Part model, mm, in its own coordinate system. A direction names the side the tool comes from. Round coordinates to 2 decimals unless told otherwise and drop trailing zeros. Loops run counter-clockwise (first coordinate to the right, second up) from the corner with the lowest first, then second, coordinate; pieces in that order, holes last. Notation, with made-up numbers: M 14.25,59 L 31.25,59 A23 ccw 31.25,93 Z; hole C -37.5,44 d1. An arc over 180 degrees is marked long. Write each question's results on one line, items separated by ' | '.
from build123d import *

# Parameters (mm, degrees)
SKETCH2_R                                       = 7.5
BOSS_EXTRUDE1_DEPTH                             = 8
CSK_FOR_M3_FLAT_HEAD_MACHINE_SCREW2_D           = 3.2
CSK_FOR_M3_FLAT_HEAD_MACHINE_SCREW2_CSINK_D     = 8.3
CSK_FOR_M3_FLAT_HEAD_MACHINE_SCREW2_CSINK_ANGLE = 90
FILLET1_R                                       = 20
V_GROOVE_CUTOUT_FLIPPED_DEPTH                   = 3.6
SKETCH49_R                                      = 2.55
CUT_EXTRUDE3_DEPTH                              = 52.922196079
CHAMFER2_SIZE                                   = 0.4
CHAMFER2_SIZE2                                  = 1.098990968
MOVE_FACE2_BY                                   = 0.5
MOVE_FACE2_2_BY                                 = 0.5
MOVE_FACE2_3_BY                                 = 0.5
MOVE_FACE2_4_BY                                 = 0.5
MOVE_FACE2_5_BY                                 = 0.5
MOVE_FACE2_6_BY                                 = 0.5
CIRPATTERN2_COUNT                               = 3
SKETCH20_R                                      = 1.375
TOOL_WING_SCREW_HOLES_DEPTH                     = 4
FILLET17_R                                      = 2
FILLET18_R                                      = 1
SKETCH50_R                                      = 1.375
CUT_EXTRUDE4_DEPTH                              = 4


with BuildPart() as part:
    # Sketch2 → Boss-Extrude1 (new body)
    with BuildSketch(Plane.XY):
        Polygon((-18, 40), (18, 40), (18, -4.618802154), (32.810889132, -13.169872981), (27.810889132, -21.830127019), (-27.810889132, -21.830127019), (-32.810889132, -13.169872981), (-18, -4.618802154), align=None)
        Circle(SKETCH2_R, mode=Mode.SUBTRACT)
    extrude(amount=BOSS_EXTRUDE1_DEPTH)

    # CSK for M3 Flat Head Machine Screw2 (through all)
    with Locations(Plane.XY.offset(8)):
        with Locations((-25.980762114, -15), (0, 30), (25.980762114, -15)):
            CounterSinkHole(CSK_FOR_M3_FLAT_HEAD_MACHINE_SCREW2_D / 2, CSK_FOR_M3_FLAT_HEAD_MACHINE_SCREW2_CSINK_D / 2, counter_sink_angle=CSK_FOR_M3_FLAT_HEAD_MACHINE_SCREW2_CSINK_ANGLE)

    # Fillet1
    fillet1_edges = [part.edges().sort_by_distance(p)[0] for p in [
        (18, -4.618802154, 4),
        (-18, -4.618802154, 4),
    ]]
    fillet(fillet1_edges, radius=FILLET1_R)

    # Sketch47 → v-groove cutout flipped (cut)
    with BuildSketch(Plane(origin=(0, 0, 0), x_dir=(-1, 0, 0), z_dir=(0, 0, -1))):
        with BuildLine():
            Line((-3.464101615, 14), (-13.856406461, -4))
            ThreePointArc((-13.856406461, -4), (-13.856406461, -8), (-10.392304845, -10))
            Line((-10.392304845, -10), (10.392304845, -10))
            ThreePointArc((10.392304845, -10), (13.856406461, -8), (13.856406461, -4))
            Line((13.856406461, -4), (3.464101615, 14))
            ThreePointArc((3.464101615, 14), (0, 16), (-3.464101615, 14))
        make_face()
    extrude(amount=-V_GROOVE_CUTOUT_FLIPPED_DEPTH, mode=Mode.SUBTRACT)

    # Sketch49 → Cut-Extrude3 (cut, through all)
    with BuildSketch(Plane(origin=(0, 0, 3.6), x_dir=(-1, 0, 0), z_dir=(0, 0, -1))):
        with Locations((0, 12)):
            Circle(SKETCH49_R)
        with Locations((10.392304845, -6)):
            Circle(SKETCH49_R)
        with Locations((-10.392304845, -6)):
            Circle(SKETCH49_R)
    extrude(amount=-CUT_EXTRUDE3_DEPTH, mode=Mode.SUBTRACT)

    # Chamfer2
    chamfer2_edges = [part.edges().sort_by_distance(p)[0] for p in [
        (2.55, 12, 8),
        (-7.842304845, -6, 8),
        (12.942304845, -6, 8),
    ]]
    chamfer2_side = [part.faces().sort_by_distance(p)[0] for p in [
        (17.098380214, 23.464101615, 8),
    ]]
    chamfer(chamfer2_edges, length=CHAMFER2_SIZE, length2=CHAMFER2_SIZE2, reference=chamfer2_side[0])

    # Move Face2: a curved face moved inward by 0.5
    add(Solid.thicken(part.faces().sort_by_distance((-13.856406461, -8, 1.8))[0], -MOVE_FACE2_BY), mode=Mode.SUBTRACT)

    # Move Face2 2: a face moved inward by 0.5
    extrude(part.faces().sort_by_distance((0, -10, 1.8))[0], amount=MOVE_FACE2_2_BY, dir=(0, -1, 0), mode=Mode.SUBTRACT)

    # Move Face2 3: a curved face moved inward by 0.5
    add(Solid.thicken(part.faces().sort_by_distance((13.856406461, -8, 1.8))[0], -MOVE_FACE2_3_BY), mode=Mode.SUBTRACT)

    # Move Face2 4: a face moved inward by 0.5
    extrude(part.faces().sort_by_distance((8.660254038, 5, 1.8))[0], amount=MOVE_FACE2_4_BY, dir=(0.866025404, 0.5, 0), mode=Mode.SUBTRACT)

    # Move Face2 5: a curved face moved inward by 0.5
    add(Solid.thicken(part.faces().sort_by_distance((0, 16, 1.8))[0], -MOVE_FACE2_5_BY), mode=Mode.SUBTRACT)

    # Move Face2 6: a face moved inward by 0.5
    extrude(part.faces().sort_by_distance((-8.660254038, 5, 1.8))[0], amount=MOVE_FACE2_6_BY, dir=(-0.866025404, 0.5, 0), mode=Mode.SUBTRACT)

    # Sketch46 → tool ball cutout (revolve, cut)
    with BuildSketch(Plane(origin=(0, 30, 0), x_dir=(1, 0, 0), z_dir=(0, 1, 0))):
        with BuildLine():
            Line((0, 4.3), (0, -3.7))
            ThreePointArc((0, -3.7), (-4, 0.3), (0, 4.3))
        make_face()
    tool_ball_cutout = revolve(axis=Axis((0, 30, 0), (0, 0, -1)), mode=Mode.SUBTRACT)

    # CirPattern2: tool ball cutout ×3 about axis
    cirpattern2_axis = Axis((0, 0, 0), (0, 0, 1))
    for i in range(1, CIRPATTERN2_COUNT):
        add(tool_ball_cutout.rotate(cirpattern2_axis, i * 360 / CIRPATTERN2_COUNT), mode=Mode.SUBTRACT)

    # Sketch20 → Tool Wing Screw Holes (cut)
    with BuildSketch(Plane(origin=(18, 0, 0), x_dir=(0, 0, -1), z_dir=(1, 0, 0))):
        with Locations(Location((-4, 19, 0), (0, 0, 90))):
            Circle(SKETCH20_R)
        with Locations(Location((-4, 32.5, 0), (0, 0, 90))):
            Circle(SKETCH20_R)
    tool_wing_screw_holes = extrude(amount=-TOOL_WING_SCREW_HOLES_DEPTH, mode=Mode.SUBTRACT)

    # Mirror2: Tool Wing Screw Holes across plane
    add(tool_wing_screw_holes.mirror(Plane(origin=(0, 0, 0), x_dir=(0, 0, 1), z_dir=(1, 0, 0))), mode=Mode.SUBTRACT)

    # Fillet17
    fillet17_edges = [part.edges().sort_by_distance(p)[0] for p in [
        (32.810889132, -13.169872981, 4),
        (27.810889132, -21.830127019, 4),
        (-27.810889132, -21.830127019, 4),
        (-32.810889132, -13.169872981, 4),
    ]]
    fillet(fillet17_edges, radius=FILLET17_R)

    # Fillet18
    fillet18_edges = [part.edges().sort_by_distance(p)[0] for p in [
        (-18, 40, 4),
        (18, 40, 4),
    ]]
    fillet(fillet18_edges, radius=FILLET18_R)

    # Sketch50 → Cut-Extrude4 (cut)
    with BuildSketch(Plane.XZ.offset(21.830127019)):
        with Locations((-15, 4)):
            Circle(SKETCH50_R)
        with Locations((15, 4)):
            Circle(SKETCH50_R)
    extrude(amount=-CUT_EXTRUDE4_DEPTH, mode=Mode.SUBTRACT)


solid = part.part
Item 1: Band-saw the part on A-A on x = 0. Give the cut face in (y, z).
Filled sheet:
outline: M -21.83,0 L -10.5,0 L -10.5,3.6 L -7.5,3.6 L -7.5,8 L -21.83,8 Z; M 7.5,3.6 L 9.45,3.6 L 9.45,6.9 L 9.05,8 L 7.5,8 Z; M 14.55,3.6 L 16.5,3.6 L 16.5,0 L 26.01,0 A4 cw 28.4,3.37 L 28.4,5.45 L 25.85,8 L 14.95,8 L 14.55,6.9 Z; M 31.6,3.37 A4 cw 33.99,0 L 40,0 L 40,8 L 34.15,8 L 31.6,5.45 Z
Item 2: Band-saw the part on B-B on y = 0. Give the cut face in (x, z).
Filled sheet:
outline: M -19.24,0 L -12.12,0 L -12.12,3.6 L -7.5,3.6 L -7.5,8 L -19.24,8 Z; M 7.5,3.6 L 12.12,3.6 L 12.12,0 L 19.24,0 L 19.24,8 L 7.5,8 Z
Item 3: Drop flat-ended pins along their axis: P1, Ø0.8, axis at y = 18.5, z = 3.5, coming from the -X side; P2, Ø1.5, axis at y = 22, z = 1, coming from the +X side; P3, Ø6, axis at x = 17, y = -14.5, coming from the -Z side; P4, Ø6, axis at x = 0, y = 12, coming from the -Z side. Give the stop position or say it passes through.
Filled sheet:
P1: x = -14 | P2: x = 18 | P3: z = 0 | P4: z = 3.6
Item 4: Band-saw the part on C-C on y = 22. Give the cut face in (x, z).
Filled sheet:
outline: M -18,0 L 18,0 L 18,8 L -18,8 Z
Item 5: Band-saw the part on D-D on y = 12. Give the cut face in (x, z), and give its area (3 significant figures).
Filled sheet:
outline: M -18,0 L -5.2,0 L -5.2,3.6 L -2.55,3.6 L -2.55,6.9 L -2.95,8 L -18,8 Z; M 2.55,3.6 L 5.2,3.6 L 5.2,0 L 18,0 L 18,8 L 2.95,8 L 2.55,6.9 Z | area: 228 mm^2
Item 6: Which spindle directions (+Z, -Z, +X, -X, +Y, -Y) get a long thin tool onto all of the face, cutting with end or side? Do faces 1 (the flat face through (-14, 32, 4)), 2 (the flat face through (-18, 23, 4)), 3 (the flat face through (14, 19, 4)), 4 (the flat face through (-30.076, -17.908, 3.944)), 5 (the flat face through (-6, -6, 3.6)). Say none if no direction does.
Filled sheet:
face 1: -X | face 2: +Z, -Z, -X, +Y | face 3: +X | face 4: +Z, -Z, -X, -Y | face 5: -Z
Item 7: Two-plate mould, pull along X, no slides. Class faces 6 (the conical face through (0.224, 31.709, 5.574)), 7 (the cylindrical face through (16.028, 31.126, 4.06)), 8 (the cylindrical face through (14.322, -8.193, 1.775)), 9 (the flat face through (-14, 19, 4)): +X half, -X half, draft (parallel to the pull), parting line (faces both ways), or undercut.
Filled sheet:
face 6: undercut | face 7: draft | face 8: undercut | face 9: -X half
Item 8: Wall check: L1, parallel to Y at x = 0, z = 4.9; L2, parallel to Y at x = -15, z = 3; L3, parallel to Z at x = -15, y = -20.25 (3 decimals). Give the ranges that are in metal, low to high.
Filled sheet:
L1: -21.83 to -7.5, 7.5 to 9.45, 14.55 to 28.4, 31.6 to 40 | L2: -17.83 to 18.06, 19.94 to 31.56, 33.44 to 40 | L3: 0 to 2.625, 5.375 to 8
